```python
from build123d import *

# Parameters (mm, degrees)
SKETCH1_W           = 3.175
SKETCH1_H           = 12.7
SKETCH2_W           = 21.844
SKETCH2_H           = 9.525
BOSS_EXTRUDE1_DEPTH = 12.827
FILLET4_R           = 1.27
SKETCH3_W           = 9.652
SKETCH3_H           = 3.175
CUT_EXTRUDE1_DEPTH  = 22.844
SKETCH4_R           = 1.5875
CUT_EXTRUDE2_DEPTH  = 10.525
FILLET5_R           = 0.762


with BuildPart() as part:
    # Sketch1 → Revolve1 (revolve)
    with BuildSketch(Plane(origin=(0, 0, 0), x_dir=(1, 0, 0), z_dir=(0, 1, 0))):
        with Locations((1.5875, 6.35)):
            Rectangle(SKETCH1_W, SKETCH1_H)
    revolve(axis=Axis((0, 0, -12.7), (0, 0, 1)))

    # Sketch2 → Boss-Extrude1 (add)
    with BuildSketch(Plane.XY):
        Rectangle(SKETCH2_W, SKETCH2_H)
    extrude(amount=BOSS_EXTRUDE1_DEPTH)

    # Fillet4
    fillet4_edges = [part.edges().sort_by_distance(p)[0] for p in [
        (10.922, -4.7625, 6.4135),
        (0, 4.7625, 0),
        (10.922, 4.7625, 6.4135),
        (-10.922, 0, 0),
        (-10.922, 4.7625, 6.4135),
        (0, -4.7625, 0),
        (-10.922, -4.7625, 6.4135),
        (10.922, 0, 0),
    ]]
    fillet(fillet4_edges, radius=FILLET4_R)

    # Sketch3 → Cut-Extrude1 (cut, through all)
    with BuildSketch(Plane.ZY.offset(10.922)):
        with Locations((8.001, 0)):
            Rectangle(SKETCH3_W, SKETCH3_H)
    extrude(amount=-CUT_EXTRUDE1_DEPTH, mode=Mode.SUBTRACT)

    # Sketch4 → Cut-Extrude2 (cut, through all)
    with BuildSketch(Plane(origin=(0, 4.7625, 0), x_dir=(1, 0, 0), z_dir=(0, 1, 0))):
        with Locations((-6.35, -8.0645)):
            Circle(SKETCH4_R)
        with Locations((6.35, -8.0645)):
            Circle(SKETCH4_R)
    extrude(amount=-CUT_EXTRUDE2_DEPTH, mode=Mode.SUBTRACT)

    # Fillet5
    fillet5_edges = [part.edges().sort_by_distance(p)[0] for p in [
        (-3.175, 0, 0),
        (-3.175, 0, -12.7),
    ]]
    fillet(fillet5_edges, radius=FILLET5_R)


solid = part.part
```
Geometry check sheet. Reference: the model listing, model coordinates, mm. A direction names the side the tool comes from. Coordinates: 2 decimals unless noted, no trailing zeros. Write each loop counter-clockwise with the first axis right and the second up, starting at its lowest first coordinate (ties: lowest second). Pieces come first, ordered by that corner, then holes. Notation, with made-up numbers: M 69.5,0.25 L 125.5,0.25 A12 ccw 125.5,10.25 Z; hole C -7,-25.75 d11. An arc over 180 degrees is marked long. Answer as a JSON object with one key per item and string values.
1. Section check C-C, the plane y = 0. Enter the section's corners in (x, z) (3 decimals), plus the area to 3 significant figures.
Answers below:
{"outline": "M -10.922,1.27 A1.27 ccw -9.652,0 L -3.937,0 A0.762 cw -3.175,-0.762 L -3.175,-11.938 A0.762 ccw -2.413,-12.7 L 2.413,-12.7 A0.762 ccw 3.175,-11.938 L 3.175,-0.762 A0.762 cw 3.937,0 L 9.652,0 A1.27 ccw 10.922,1.27 L 10.922,3.175 L -10.922,3.175 Z", "area": "149 mm²"}
2. Section check D-D, the plane z = 9. Enter the section's corners in (x, y), plus the area to 3 significant figures.
Answers below:
{"outline": "M -10.92,-3.49 A1.27 ccw -9.65,-4.76 L -7.63,-4.76 L -7.63,-1.59 L -10.92,-1.59 Z; M -10.92,1.59 L -7.63,1.59 L -7.63,4.76 L -9.65,4.76 A1.27 ccw -10.92,3.49 Z; M -5.07,-4.76 L 5.07,-4.76 L 5.07,-1.59 L -5.07,-1.59 Z; M -5.07,1.59 L 5.07,1.59 L 5.07,4.76 L -5.07,4.76 Z; M 7.63,-4.76 L 9.65,-4.76 A1.27 ccw 10.92,-3.49 L 10.92,-1.59 L 7.63,-1.59 Z; M 7.63,1.59 L 10.92,1.59 L 10.92,3.49 A1.27 ccw 9.65,4.76 L 7.63,4.76 Z", "area": "105 mm²"}
3. Section check A-A, the plane z = 4.5. Enter the section's corners in (x, y), plus the area to 3 significant figures.
Answers below:
{"outline": "M -10.92,-3.49 A1.27 ccw -9.65,-4.76 L 9.65,-4.76 A1.27 ccw 10.92,-3.49 L 10.92,-1.59 L -10.92,-1.59 Z; M -10.92,1.59 L 10.92,1.59 L 10.92,3.49 A1.27 ccw 9.65,4.76 L -9.65,4.76 A1.27 ccw -10.92,3.49 Z", "area": "137 mm²"}
4. Section check B-B, the plane x = -6.35. Enter the section's corners in (y, z) (1 decimal), plus the area to 3 significant figures.
Answers below:
{"outline": "M -4.8,1.3 A1.3 ccw -3.5,0 L 3.5,0 A1.3 ccw 4.8,1.3 L 4.8,6.5 L 1.6,6.5 L 1.6,3.2 L -1.6,3.2 L -1.6,6.5 L -4.8,6.5 Z; M -4.8,9.7 L -1.6,9.7 L -1.6,12.8 L -4.8,12.8 Z; M 1.6,9.7 L 4.8,9.7 L 4.8,12.8 L 1.6,12.8 Z", "area": "70.7 mm²"}
5. Scan lines: L1, parallel to Y at x = 2.75, z = 9.25; L2, parallel to Z at x = -6.35, y = 2.5; L3, parallel to Z at x = 4, y = -0.25 (3 decimals). Record each from-to range of solid material in increasing order.
Answers below:
{"L1": "y = -4.76 to -1.59, 1.59 to 4.76", "L2": "z = 0 to 6.48, 9.65 to 12.83", "L3": "z = 0 to 3.175"}
6. Go/stop test with flat-tipped pins: pin 1 Ø3 at (x, z) = (6.35, 8.06) entering from +Y; pin 2 Ø2 at (x, y) = (-5.5, -1.5) entering from -Z. Record where each tip stops, or that it passes through.
Answers below:
{"pin 1": "passes through", "pin 2": "stops at z = 0"}
7. Draft check along Z on faces 1 (the flat face through (0, 1.588, 8)), 2 (the cylindrical face through (6.14, 3.2, 6.49)), 3 (the cylindrical face through (0.14, -4.4, 0.38)). Enter one of: released by +Z, released by -Z, zero draft, split by the parting line, or undercut.
Answers below:
{"face 1": "zero draft", "face 2": "undercut", "face 3": "released by -Z"}
8. Tool access check on faces 4 (the cylindrical face through (10.54, 4.4, 7.13)), 5 (the flat face through (0, -1.588, 8)). Record the directions out of +Z, -Z, +X, -X, +Y, -Y that give a thin tool (end or side, any length) a straight path to the whole face; none if there is none.
Answers below:
{"face 4": "+Z, -Z, +X, +Y", "face 5": "+Z, +X, -X"}
